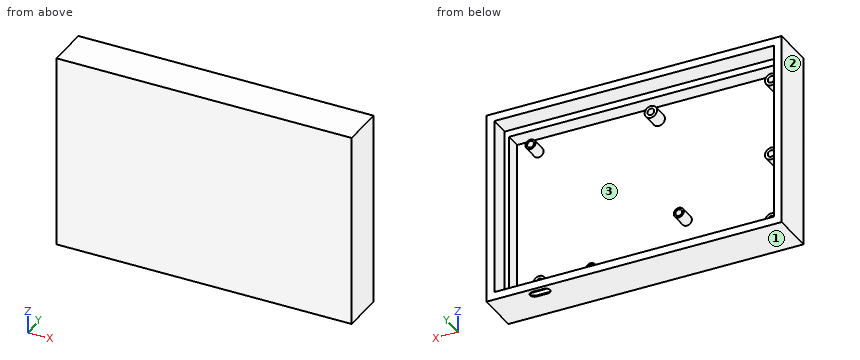
```python
from build123d import *

# Parameters (mm, degrees)
SKETCH1_W           = 125
SKETCH1_H           = 80
BOSS_EXTRUDE1_DEPTH = 3
SKETCH1_3_W         = 132
SKETCH1_3_H         = 87
SKETCH1_3_W_2       = 125
SKETCH1_3_H_2       = 80
BOSS_EXTRUDE2_DEPTH = 19
SKETCH2_W           = 125
SKETCH2_H           = 80
SKETCH2_W_2         = 120
SKETCH2_H_2         = 76
BOSS_EXTRUDE3_DEPTH = 10
SKETCH3_W           = 28.6783421
SKETCH3_H           = 5.698707123
CUT_EXTRUDE1_DEPTH  = 3
CUT_EXTRUDE2_DEPTH  = 3
SKETCH5_R           = 2.75
SKETCH5_R_2         = 1.5
SKETCH5_R_3         = 2.259305414
BOSS_EXTRUDE4_DEPTH = 7


with BuildPart() as part:
    # Sketch1 → Boss-Extrude1 (new body)
    with BuildSketch(Plane(origin=(0, 0, 0), x_dir=(1, 0, 0), z_dir=(0, 1, 0))):
        Rectangle(SKETCH1_W, SKETCH1_H)
    extrude(amount=BOSS_EXTRUDE1_DEPTH)

    # Sketch1_3 → Boss-Extrude2 (add)
    with BuildSketch(Plane(origin=(0, 0, 0), x_dir=(1, 0, 0), z_dir=(0, 1, 0))):
        Rectangle(SKETCH1_3_W, SKETCH1_3_H)
        Rectangle(SKETCH1_3_W_2, SKETCH1_3_H_2, mode=Mode.SUBTRACT)
    extrude(amount=BOSS_EXTRUDE2_DEPTH)

    # Sketch2 → Boss-Extrude3 (add)
    with BuildSketch(Plane(origin=(0, 0, 0), x_dir=(1, 0, 0), z_dir=(0, 1, 0))):
        Rectangle(SKETCH2_W, SKETCH2_H)
        with Locations((0.5, 1)):
            Rectangle(SKETCH2_W_2, SKETCH2_H_2, mode=Mode.SUBTRACT)
    extrude(amount=BOSS_EXTRUDE3_DEPTH)

    # Sketch3 → Cut-Extrude1 (cut)
    with BuildSketch(Plane(origin=(0, 0, -40), x_dir=(-1, 0, 0), z_dir=(0, 0, -1))):
        with Locations((-43.918315426, 14.566401795)):
            Rectangle(SKETCH3_W, SKETCH3_H)
    extrude(amount=CUT_EXTRUDE1_DEPTH, mode=Mode.SUBTRACT)

    # Sketch4 → Cut-Extrude2 (cut)
    with BuildSketch(Plane(origin=(0, 0, -43.5), x_dir=(-1, 0, 0), z_dir=(0, 0, -1))):
        with BuildLine():
            Line((-46.454793207, 17.25655779), (-41.357520978, 17.25655779))
            ThreePointArc((-41.357520978, 17.25655779), (-39.417949113, 15.316985924), (-41.357520978, 13.377414059))
            Line((-41.357520978, 13.377414059), (-46.454793207, 13.377414059))
            ThreePointArc((-46.454793207, 13.377414059), (-48.394365073, 15.316985924), (-46.454793207, 17.25655779))
        make_face()
    extrude(amount=-CUT_EXTRUDE2_DEPTH, mode=Mode.SUBTRACT)

    # Sketch5 → Boss-Extrude4 (add)
    # profile 1 of 8: a face of its own
    with BuildSketch(Plane(origin=(0, 3, 0), x_dir=(1, 0, 0), z_dir=(0, 1, 0))):
        with Locations(Location((-56.666408857, -30.772899219, 0), (0, 0, 90))):
            Circle(SKETCH5_R)
        with Locations(Location((-56.666408857, -30.772899219, 0), (0, 0, 270))):
            Circle(SKETCH5_R_2, mode=Mode.SUBTRACT)
    # profile 2 of 8: a face of its own
    with BuildSketch(Plane(origin=(0, 3, 0), x_dir=(1, 0, 0), z_dir=(0, 1, 0))):
        with Locations(Location((-56.666408857, 34.623451832, 0), (0, 0, 90))):
            Circle(SKETCH5_R)
        with Locations(Location((-56.666408857, 34.623451832, 0), (0, 0, 270))):
            Circle(SKETCH5_R_2, mode=Mode.SUBTRACT)
    # profile 3 of 8: a face of its own
    with BuildSketch(Plane(origin=(0, 3, 0), x_dir=(1, 0, 0), z_dir=(0, 1, 0))):
        with Locations(Location((-56.666408857, 3.874879483, 0), (0, 0, 90))):
            Circle(SKETCH5_R)
        with Locations(Location((-56.666408857, 3.874879483, 0), (0, 0, 270))):
            Circle(SKETCH5_R_2, mode=Mode.SUBTRACT)
    # profile 4 of 8: a face of its own
    with BuildSketch(Plane(origin=(0, 3, 0), x_dir=(1, 0, 0), z_dir=(0, 1, 0))):
        with Locations(Location((-15.376408857, 19.879433801, 0), (0, 0, 90))):
            Circle(SKETCH5_R_3)
        with Locations(Location((-15.376408857, 19.879433801, 0), (0, 0, 270))):
            Circle(SKETCH5_R_2, mode=Mode.SUBTRACT)
    # profile 5 of 8: a face of its own
    with BuildSketch(Plane(origin=(0, 3, 0), x_dir=(1, 0, 0), z_dir=(0, 1, 0))):
        with Locations(Location((24.041591143, 34.623451832, 0), (0, 0, 90))):
            Circle(SKETCH5_R_3)
        with Locations(Location((24.041591143, 34.623451832, 0), (0, 0, 270))):
            Circle(SKETCH5_R_2, mode=Mode.SUBTRACT)
    # profile 6 of 8: a face of its own
    with BuildSketch(Plane(origin=(0, 3, 0), x_dir=(1, 0, 0), z_dir=(0, 1, 0))):
        with Locations(Location((50.940615446, -30.772899219, 0), (0, 0, 90))):
            Circle(SKETCH5_R_3)
        with Locations(Location((50.940615446, -30.772899219, 0), (0, 0, 270))):
            Circle(SKETCH5_R_2, mode=Mode.SUBTRACT)
    # profile 7 of 8: a face of its own
    with BuildSketch(Plane(origin=(0, 3, 0), x_dir=(1, 0, 0), z_dir=(0, 1, 0))):
        with Locations(Location((-2.862896706, -30.772899219, 0), (0, 0, 90))):
            Circle(SKETCH5_R)
        with Locations(Location((-2.862896706, -30.772899219, 0), (0, 0, 270))):
            Circle(SKETCH5_R_2, mode=Mode.SUBTRACT)
    # profile 8 of 8: a face of its own
    with BuildSketch(Plane(origin=(0, 3, 0), x_dir=(1, 0, 0), z_dir=(0, 1, 0))):
        with Locations(Location((47.016763874, 34.623451832, 0), (0, 0, 90))):
            Circle(SKETCH5_R)
        with Locations(Location((47.016763874, 34.623451832, 0), (0, 0, 270))):
            Circle(SKETCH5_R_2, mode=Mode.SUBTRACT)
    extrude(amount=BOSS_EXTRUDE4_DEPTH)


solid = part.part
```
Input: part model. Units: mm. Frame: model coordinates. Face numbers are marked on the shaded views. Coordinates: 2 decimals unless noted, no trailing zeros. Order: outer loops, then holes, each group sorted by start corner. A loop starts at its lowest first (then second) coordinate and runs counter-clockwise, first axis right, second up. Notation, with made-up numbers: (50.25, 78) - (84.25, 78) arc R14 ccw to (84.25, 95) - close; hole circle Ø7 at (-27.5, -21). An arc over 180 degrees is marked (long way). Put each result on its own line as item: value.
1. Contact query for flat-ended pins moving along their axis: pin 1 Ø6 at (x, z) = (-56.5, 31) entering from +Y; pin 2 Ø1.5 at (x, z) = (-56, 31) entering from +Y. Output: stop coordinate, or through.
Report:
pin 1: stops at y = 10
pin 2: stops at y = 3
2. Cut plane A-A on y = 8.5. State how many separate pieces and enclosed holes the cut face has, then the cut area to 3 significant figures.
Report:
separate pieces: 9
enclosed holes: 9
area: 2,470 mm2
3. Cut plane B-B on x = -51.5. Return the cut outline in (y, z), then the cut area to 3 significant figures.
Report:
outline: (0, -43.5) - (19, -43.5) - (19, -40) - (10, -40) - (10, -39) - (3, -39) - (3, 37) - (10, 37) - (10, 40) - (19, 40) - (19, 43.5) - (0, 43.5) - close
area: 401 mm2
4. Draft query along X for the marked faces 1, 2 and 3. Return one class per face: pulls with the +X half, pulls with the -X half, needs draft (parallel to the pull), parting line crosses it, or undercut.
Report:
face 1: needs draft
face 2: pulls with the -X half
face 3: undercut
5. Cut plane C-C on z = 7.5. Return the cut outline in (x, y), then the cut area to 3 significant figures.
Report:
outline: (-66, 0) - (66, 0) - (66, 19) - (62.5, 19) - (62.5, 10) - (60.5, 10) - (60.5, 3) - (-59.5, 3) - (-59.5, 10) - (-62.5, 10) - (-62.5, 19) - (-66, 19) - close
area: 543 mm2
6. Cut plane D-D on y = 15.5. Return the cut outline in (x, z).
Report:
outline: (-66, -43.5) - (39.43, -43.5) - (39.43, -43) - (29.58, -43) - (29.58, -40) - (-62.5, -40) - (-62.5, 40) - (62.5, 40) - (62.5, -40) - (58.26, -40) - (58.26, -43) - (48.39, -43) - (48.39, -43.5) - (66, -43.5) - (66, 43.5) - (-66, 43.5) - close
7. Line query: line 1 along X through (y, z) = (15.25, -37.5); line 2 along Z through (x, y) = (-27, 11); line 3 along Z through (x, y) = (-16, 8.5). Output: solid intervals per line, ascending.
Report:
line 1: x = -66 to -62.5, 62.5 to 66
line 2: z = -43.5 to -40, 40 to 43.5
line 3: z = -43.5 to -39, -22.05 to -21.24, -18.52 to -17.71, 37 to 43.5
